from build123d import *

# Parameters (mm, degrees)
F0_W           = 12.7
F0_H           = 12.7
F0_H_2         = 38.1
F0_W_2         = 76.2
F1_DEPTH       = 7.62
F2_DEPTH       = 12.7
F3_DEPTH       = 76.2
F5_DEPTH       = 6.35
F6_W           = 1.980378
F6_H           = 38.16213
F7_DEPTH       = 76.2
F9_DEPTH       = 47.752
F9_DEPTH_BACK  = 50.292
F10_DEPTH      = 47.752
F10_DEPTH_BACK = 50.292
F11_W          = 1.980378
F11_H          = 68.58
F12_DEPTH      = 1.27
F12_DEPTH_BACK = 39.37
F14_DEPTH      = 90.17
F15_DEPTH      = 90.424
F16_W          = 7.112
F16_H          = 6.043921
F17_DEPTH      = 97.028


with BuildPart() as f1:
    # F0 (on Top) → F1 (new body)
    with BuildSketch(Plane.XY):
        with Locations((-57.942608, 57.15)):
            Rectangle(F0_W, F0_H)
        with Locations((-57.942608, 31.75)):
            Rectangle(F0_W, F0_H_2)
        with Locations((-57.942608, 6.35)):
            Rectangle(F0_W, F0_H)
        with Locations((-13.492608, 6.35)):
            Rectangle(F0_W_2, F0_H)
        with Locations((30.957392, 6.35)):
            Rectangle(F0_W, F0_H)
        with Locations((30.957392, 31.75)):
            Rectangle(F0_W, F0_H_2)
        with Locations((30.957392, 57.15)):
            Rectangle(F0_W, F0_H)
        with Locations((-13.492608, 57.15)):
            Rectangle(F0_W_2, F0_H)
    extrude(amount=F1_DEPTH)

    # F0 (on Top) → F2 (join)
    with BuildSketch(Plane.XY):
        with Locations((-57.942608, 6.35)):
            Rectangle(F0_W, F0_H)
        with Locations((-57.942608, 57.15)):
            Rectangle(F0_W, F0_H)
        with Locations((30.957392, 57.15)):
            Rectangle(F0_W, F0_H)
        with Locations((30.957392, 6.35)):
            Rectangle(F0_W, F0_H)
    extrude(amount=-F2_DEPTH)

    # F0 (on Top) → F3 (join)
    with BuildSketch(Plane.XY):
        with Locations((30.957392, 6.35)):
            Rectangle(F0_W, F0_H)
        with Locations((30.957392, 57.15)):
            Rectangle(F0_W, F0_H)
        with Locations((-57.942608, 57.15)):
            Rectangle(F0_W, F0_H)
        with Locations((-57.942608, 6.35)):
            Rectangle(F0_W, F0_H)
    extrude(amount=F3_DEPTH)

    # F4 (on face) → F5 (join)
    with BuildSketch(Plane.XY.offset(76.2)):
        Polygon((-64.292608, 63.5), (-64.292608, -88.9), (37.307392, -88.9), (37.307392, 63.5), (37.307392, 114.3), (-64.292608, 114.3), align=None)
    extrude(amount=F5_DEPTH)

    # F6 (on face) → F7 (join)
    with BuildSketch(Plane(origin=(0, 0, 76.2), x_dir=(1, 0, 0), z_dir=(0, 0, -1))):
        with Locations((-12.502419, -31.781065)):
            Rectangle(F6_W, F6_H)
    extrude(amount=F7_DEPTH)

    # F8 (on face) → F9 (join, two sides)
    with BuildSketch(Plane.YZ.offset(-11.51223)) as f9_sk:
        Polygon((30.57342, 41.91), (12.7, 41.91), (12.7, 9.275453), (50.86213, 9.275453), (50.86213, 41.91), (33.018019, 41.91), (33.018019, 39.962422), (30.57342, 39.962422), align=None)
    extrude(amount=F9_DEPTH)
    extrude(f9_sk.sketch, amount=-F9_DEPTH_BACK)

    # F8 (on face) → F10 (join, two sides)
    with BuildSketch(Plane.YZ.offset(-11.51223)) as f10_sk:
        Polygon((30.57342, 75.306833), (12.7, 75.306833), (12.7, 43.47302), (50.86213, 43.47302), (50.86213, 75.306833), (33.018019, 75.306833), (33.018019, 73.520184), (30.57342, 73.520184), align=None)
    extrude(amount=F10_DEPTH)
    extrude(f10_sk.sketch, amount=-F10_DEPTH_BACK)

    # F11 (on face) → F12 (join, two sides)
    with BuildSketch(Plane(origin=(0, 50.86213, 0), x_dir=(-1, 0, 0), z_dir=(0, 1, 0))) as f12_sk:
        with Locations((12.502419, 41.91)):
            Rectangle(F11_W, F11_H)
    extrude(amount=F12_DEPTH)
    extrude(f12_sk.sketch, amount=-F12_DEPTH_BACK)

    # F13 (on face) → F14 (join)
    with BuildSketch(Plane(origin=(0, 0, 76.2), x_dir=(1, 0, 0), z_dir=(0, 0, -1))):
        Polygon((-16.877052, 79.53029), (-20.790081, 85.46904), (-26.72883, 81.556011), (-22.815801, 75.617261), align=None)
    extrude(amount=F14_DEPTH)

    # F13 (on face) → F15 (join)
    with BuildSketch(Plane(origin=(0, 0, 76.2), x_dir=(1, 0, 0), z_dir=(0, 0, -1))):
        Polygon((-16.877052, 79.53029), (-20.790081, 85.46904), (-26.72883, 81.556011), (-22.815801, 75.617261), align=None)
    extrude(amount=F15_DEPTH)

    # F16 (on face) → F17 (join)
    with BuildSketch(Plane(origin=(-41.648083, -63.208712, 0), x_dir=(-0.835032, 0.550201, 0), z_dir=(0.550201, 0.835032, 0))):
        with Locations((-26.108759, 10.307214)):
            Rectangle(F16_W, F16_H)
    extrude(amount=F17_DEPTH)


solid = f1.part
Verification items for the finished model (mm, model axes). A direction names the side the tool comes from. Give positions to 0.01 mm unless a question says otherwise; leave off trailing zeros. Write each loop counter-clockwise with the first axis right and the second up, starting at its lowest first coordinate (ties: lowest second). Pieces come first, ordered by that corner, then holes. Notation, with made-up numbers: M 31.25,33.25 L 68.25,33.25 A23 ccw 68.25,64.25 Z; hole C 11,26.5 d8. An arc over 180 degrees is marked long. Put each result on its own line as item: value. Start each with the question number.
1. Go/stop test with flat-tipped pins: pin 1 Ø12 at (x, z) = (-48, 39.5) entering from -Y; pin 2 Ø12 at (x, y) = (16, 92) entering from -Z; pin 3 Ø2.5 at (x, z) = (-23.5, 5) entering from -Y. Record where each tip stops, or that it passes through.
2. Draft check along Y on faces 1 (the face through (37, 12.7, 32)), 2 (the face through (-13, 114.3, 79)), 3 (the face through (37.307, 12, 49)). Enter one of: +Y half, -Y half, draft (parallel to the pull), parting line (faces both ways), or undercut.
3. Section check C-C (y = 21.5). Give the number of separate pieces and of enclosed holes in the cut face, and give its area (3 significant figures).
4. Set-up check for faces 4 (the face through (-33, 12.7, 26)), 5 (the face through (24.607, 57, 41)), 6 (the face through (-58, 50.8, -6)), 7 (the face through (-37, 22, 75.307)), 8 (the face through (-51.593, 6, 41)): record each of +Z, -Z, +X, -X, +Y, -Y from which the full face is reachable in a straight line by a thin tool's end or side.
5. Section check B-B (x = -49.5). Record the cut outline in (y, z).
6. Scan lines: line 1 along Z through (x, y) = (-8.5, 28); line 2 along Y through (x, z) = (-49.5, 2); line 3 along X through (y, z) = (5, 73). Record each from-to range of solid material in increasing order. Write a range as [from, to].
7. Section check A-A (z = 2). Record the cut outline in (x, y), and give its area (3 significant figures).
Answer list:
1. pin 1: y = 0
1. pin 2: z = 76.2
1. pin 3: y = -84.51
2. face 1: undercut
2. face 2: +Y half
2. face 3: draft
3. separate pieces: 3
3. enclosed holes: 0
3. area: 7,180 mm2
4. face 4: none
4. face 5: +Y
4. face 6: -Z, +X, -X
4. face 7: -X
4. face 8: -Y
5. outline: M -88.9,76.2 L 114.3,76.2 L 114.3,82.55 L -88.9,82.55 Z; M 0,0 L 12.7,0 L 12.7,7.62 L 0,7.62 Z; M 12.7,9.28 L 50.86,9.28 L 50.86,41.91 L 33.02,41.91 L 33.02,39.96 L 30.57,39.96 L 30.57,41.91 L 12.7,41.91 Z; M 12.7,43.47 L 50.86,43.47 L 50.86,75.31 L 33.02,75.31 L 33.02,73.52 L 30.57,73.52 L 30.57,75.31 L 12.7,75.31 Z; M 50.8,0 L 63.5,0 L 63.5,7.62 L 50.8,7.62 Z
6. line 1: [9.28, 41.91], [43.47, 75.31], [76.2, 82.55]
6. line 2: [0, 12.7], [50.8, 63.5]
6. line 3: [-64.29, -51.59], [24.61, 37.31]
7. outline: M -64.29,0 L 37.31,0 L 37.31,63.5 L -64.29,63.5 Z; M -26.73,-81.56 L -20.79,-85.47 L -16.88,-79.53 L -22.82,-75.62 Z; hole M -51.59,12.7 L -13.49,12.7 L -13.49,50.8 L -51.59,50.8 Z; hole M -11.51,12.7 L 24.61,12.7 L 24.61,50.8 L -11.51,50.8 Z
7. area: 3,670 mm2
